Autodesk Inventor part; units mm, degrees
ref_plane "YZ Plane" through (0, 0, 0) normal (1, 0, 0) x (0, 1, 0)
ref_plane "XZ Plane" through (0, 0, 0) normal (0, 1, 0) x (-1, 0, 0)
ref_plane "XY Plane" through (0, 0, 0) normal (0, 0, 1) x (1, 0, 0)
sketch "Esquisse1" plane through (0, 0, 0) normal (0, 0, 1) x (1, 0, 0)
  line L0 (-954.3902, 760.3659) -> (765.6098, 760.3659)
  line L1 (765.6098, 760.3659) -> (765.6098, -1389.6341)
  line L2 (765.6098, -1389.6341) -> (-954.3902, -1389.6341)
  line L3 (-954.3902, -1389.6341) -> (-954.3902, 760.3659)
  point P0 (0, 0)
  dimension "d0" = 1720
  dimension "d1" = 2150
extrude "Extrusion1" add sketch "Esquisse1" along normal blind 860
sketch "Esquisse2" plane through (-954.3902, 760.3659, 0) normal (0, 1, 0) x (1, 0, 0)
  line L0 (1720, -860) -> (0, -860)
  line L1 (40, -860) -> (1680, -860)
  line L2 (1680, -860) -> (1680, -200)
  line L3 (1680, -200) -> (40, -200)
  line L4 (40, -200) -> (40, -860)
  line L5 (0, 0) -> (1720, 0)
  point P0 (954.3902, 0)
  dimension "d4" = 40
  dimension "d5" = 40
  dimension "d6" = 200
extrude "Extrusion2" cut sketch "Esquisse2" against normal through all
sketch "Esquisse3" plane through (-914.3902, 760.3659, 200) normal (0, 0, 1) x (1, 0, 0)
  line L0 (0, -2150) -> (0, 0)
  line L1 (1640, 0) -> (1640, -2150)
  line L2 (0, -50) -> (1640, -50)
  line L3 (1640, -50) -> (1640, -2150)
  line L4 (1640, -2150) -> (0, -2150)
  line L5 (0, -2150) -> (0, -50)
  line L6 (0, 0) -> (1640, 0)
  point P0 (914.3902, -760.3659)
  dimension "d9" = 50
extrude "Extrusion3" cut sketch "Esquisse3" against normal blind 1000 contours L0 L2 L1 L4
properties part number "Porte Double" material "Bois (Chêne)"
Here's how the part is built. I have some questions about the finished solid (model axes, mm). A direction names the side the tool comes from. Coordinates: 2 decimals unless noted, no trailing zeros. Order: outer loops, then holes, each group sorted by start corner. A loop starts at its lowest first (then second) coordinate and runs counter-clockwise, first axis right, second up.
Item 1: If we section it at B-B, the plane y = -398.5: List the corners of the cut face in (x, z) for me.
Response values:
outline: (-954.39, 0) - (-914.39, 0) - (-914.39, 860) - (-954.39, 860) - close; (725.61, 0) - (765.61, 0) - (765.61, 860) - (725.61, 860) - close
Item 2: If we section it at C-C, the plane z = 171: List the corners of the cut face in (x, y) for me, then the cut area to 3 significant figures.
Response values:
outline: (-954.39, -1389.63) - (-914.39, -1389.63) - (-914.39, 710.37) - (725.61, 710.37) - (725.61, -1389.63) - (765.61, -1389.63) - (765.61, 760.37) - (-954.39, 760.37) - close
area: 254,000 mm2
Item 3: If we section it at A-A, the plane z = 716.5: List the corners of the cut face in (x, y) for me.
Response values:
outline: (-954.39, -1389.63) - (-914.39, -1389.63) - (-914.39, 760.37) - (-954.39, 760.37) - close; (725.61, -1389.63) - (765.61, -1389.63) - (765.61, 760.37) - (725.61, 760.37) - close
Item 4: Thinking about a two-plate mould opening in X: for faces 1 (the face through (-98, 760.366, 141)), 2 (the face through (765.61, -300, 424)), 3 (the face through (-106, 710.366, 101)), which applies, pulls with the +X half, pulls with the -X half, needs draft (parallel to the pull), parting line crosses it, or undercut?
Response values:
face 1: needs draft
face 2: pulls with the +X half
face 3: undercut
Item 5: I need wall thicknesses on probe 1 along X at (y, z) = (-750.5, 239); probe 2 along Y at (x, z) = (-302, 162). Which ranges of each line are inside material? Lowest first, please.
Response values:
probe 1: x = -954.39 to -914.39, 725.61 to 765.61
probe 2: y = 710.37 to 760.37
Item 6: Which directions (+Z, -Z, +X, -X, +Y, -Y) give clear straight access to the entire face, cutting with the end or side of a thin tool? Please do faces 4 (the face through (-954.39, -330, 424)), 5 (the face through (-83, 736, 200)).
Response values:
face 4: +Z, -Z, -X, +Y, -Y
face 5: +Z, +Y, -Y
Item 7: If we section it at D-D, the plane x = 614.5: List the corners of the cut face in (y, z) for me, then the cut area to 3 significant figures.
Response values:
outline: (710.37, 0) - (760.37, 0) - (760.37, 200) - (710.37, 200) - close
area: 10,000 mm2
